Drawing for the job (mm, zero at the part's lowest x, y, z). Give positions to 0.01 mm unless a question says otherwise; leave off trailing zeros. Write each loop counter-clockwise with the first axis right and the second up, starting at its lowest first coordinate (ties: lowest second). Pieces come first, ordered by that corner, then holes.
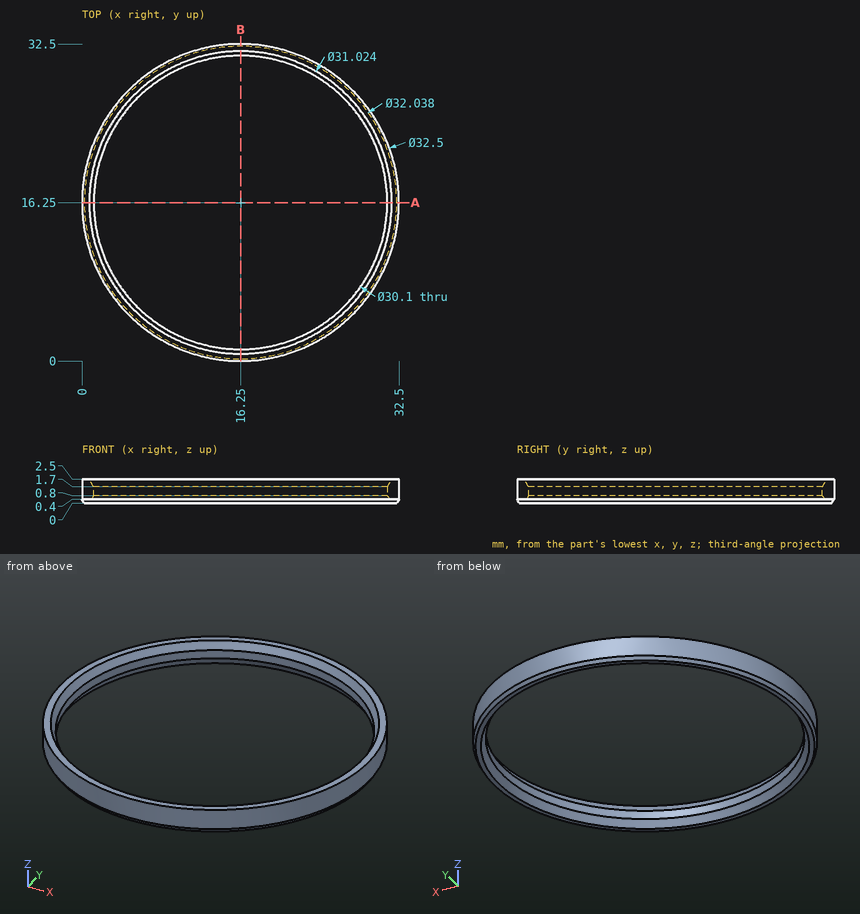
1. Pin check, flat tip, straight feed: P1, Ø1, axis at x = 13.5, z = 2, coming from the -Y side. Stop position of the tip, or through.
Calculated:
P1: stops at y = 0.16
2. Slice it at A-A, the plane y = 16.25. Write the cut outline in (x, z).
Calculated:
outline: (0, 0.4) - (0.23, 0) - (0.74, 0) - (1.2, 0.8) - (1.2, 1.7) - (0.74, 2.5) - (0, 2.5) - close; (31.3, 0.8) - (31.76, 0) - (32.27, 0) - (32.5, 0.4) - (32.5, 2.5) - (31.76, 2.5) - (31.3, 1.7) - close
3. Probe probe 1 along Y at (x, z) = (16.25, 1.15); probe 2 along Y at (x, z) = (30, 1.75); probe 3 along X at (y, z) = (29, 2.15) (1 decimal). List the from-to ranges inside material, lowest first.
Calculated:
probe 1: y = 0 to 1.2, 31.3 to 32.5
probe 2: y = 7.59 to 10.06, 22.44 to 24.91
probe 3: x = 6.2 to 7.8, 24.7 to 26.3
